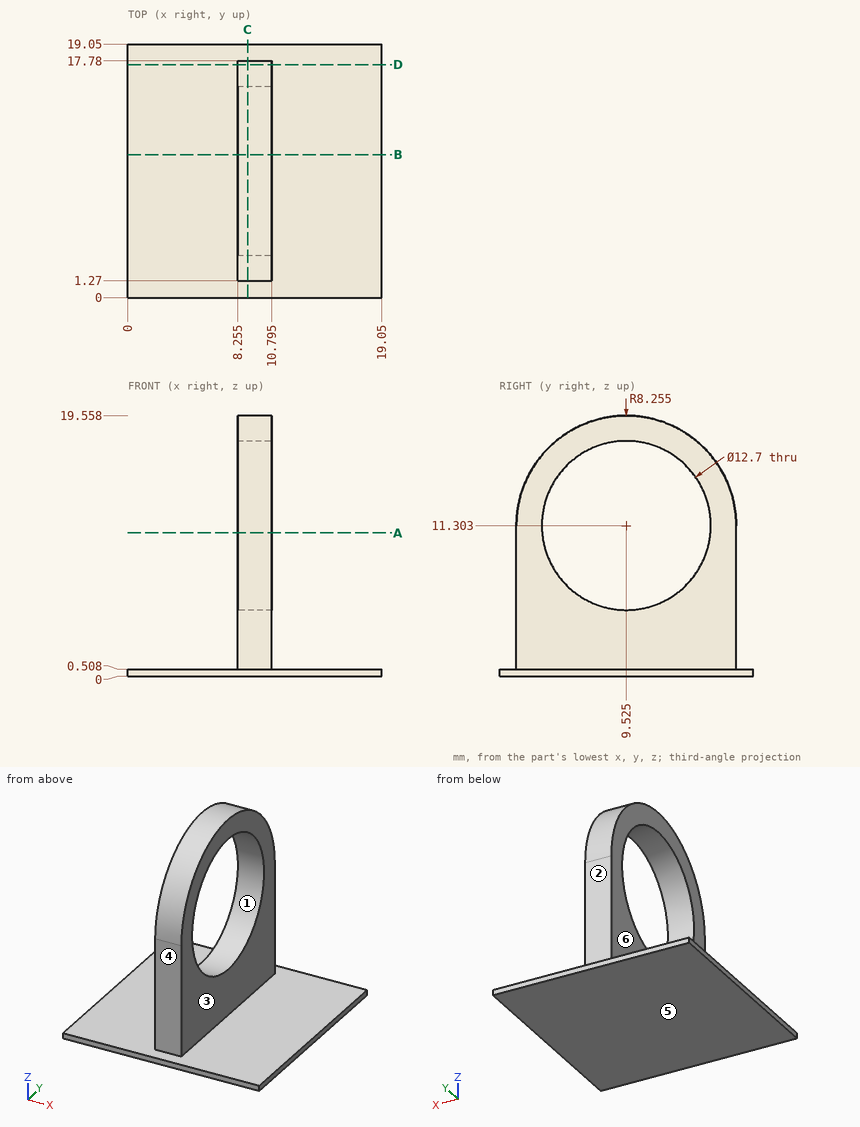
Part print with two shaded views. Sizes in mm from the minimum x, y, z corner. A direction names the side the tool comes from. Round coordinates to 2 decimals unless told otherwise and drop trailing zeros. Order: outer loops, then holes, each group sorted by start corner. A loop starts at its lowest first (then second) coordinate and runs counter-clockwise, first axis right, second up. Notation, with made-up numbers: M 3.25,48 L 27.25,48 A25 cw 27.25,74 Z; hole C -28.5,50 d3. An arc over 180 degrees is marked long. Answer in a Markdown table with one row per item. Add a question column.
Q1. 3-axis set-ups, long thin cutter, end or side, ignore diameter. For the marked faces 5 and 6: which of +Z, -Z, +X, -X, +Y, -Y reach the whole face in a straight line?
Q2. Cut at C-C on x = 9. Give the cut face in (y, z) (3 decimals).
Q3. Pin check, flat tips, straight feed: pin 1 (0.8 mm diameter, centred on x = 10, z = 3.5, fed in from +Y); pin 2 (5 mm diameter, centred on y = 6.5, z = 7, fed in from +X) (3 decimals); pin 3 (9.5 mm diameter, centred on x = 5, y = 5, fed in from +Z). Stop position of each tip, or through.
Q4. Wall check: L1, parallel to Z at x = 6.25, y = 5.5; L2, parallel to Y at x = 9, z = 13.5; L3, parallel to X at y = 8.75, z = 4.75 (3 decimals). Give the ranges that are in metal, low to high. Write a range as from..to.
Q5. Cut at D-D on y = 17.5. Give the cut face in (x, z) (3 decimals).
Q6. Cut at A-A on z = 10.75. Give the cut face in (x, y) (3 decimals), and give its area (3 significant figures).
Q7. Cut at B-B on y = 10.75. Give the cut face in (x, z) (3 decimals).
Q8. Mould opens along Y. For the marked faces 1, 2, 3 and 4 say: +Y half, -Y half, draft (parallel to the pull), parting line (faces both ways), or undercut.
Established:
| question | item | result |
|---|---|---|
| 1 | face 5 | -Z, +X, -X, +Y, -Y |
| 1 | face 6 | +Z, -X, +Y, -Y |
| 2 | outline | M 0,0 L 19.05,0 L 19.05,0.508 L 17.78,0.508 L 17.78,11.303 A8.255 ccw 1.27,11.303 L 1.27,0.508 L 0,0.508 Z; hole C 9.525,11.303 d12.7 |
| 3 | pin 1 | stops at y = 17.78 |
| 3 | pin 2 | stops at x = 10.795 |
| 3 | pin 3 | stops at z = 19.49 |
| 4 | L1 | z = 0..0.51 |
| 4 | L2 | y = 1.57..3.57, 15.48..17.48 |
| 4 | L3 | x = 8.255..10.795 |
| 5 | outline | M 0,0 L 19.05,0 L 19.05,0.508 L 10.795,0.508 L 10.795,13.435 L 8.255,13.435 L 8.255,0.508 L 0,0.508 Z |
| 6 | outline | M 8.255,1.27 L 10.795,1.27 L 10.795,3.199 L 8.255,3.199 Z; M 8.255,15.851 L 10.795,15.851 L 10.795,17.78 L 8.255,17.78 Z |
| 6 | area | 9.80 mm2 |
| 7 | outline | M 0,0 L 19.05,0 L 19.05,0.508 L 10.795,0.508 L 10.795,5.072 L 8.255,5.072 L 8.255,0.508 L 0,0.508 Z; M 8.255,17.534 L 10.795,17.534 L 10.795,19.467 L 8.255,19.467 Z |
| 8 | face 1 | undercut |
| 8 | face 2 | +Y half |
| 8 | face 3 | draft |
| 8 | face 4 | -Y half |
